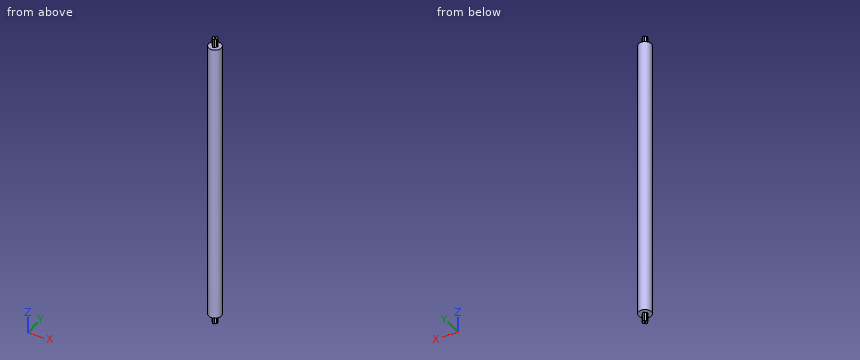
```python
from build123d import *

# Parameters (mm, degrees)
F0_R     = 22.5
F1_DEPTH = 1000
F4_DEPTH = 31
F5_R     = 2.5
F6_DEPTH = 40
F7_DEPTH = 30
F8_R     = 2.5
F9_DEPTH = 30


with BuildPart() as f1:
    # F0 (on Top) → F1 (new body)
    with BuildSketch(Plane.XY):
        Circle(F0_R)
    extrude(amount=F1_DEPTH)

    # F3 (on face) → F4 (join)
    with BuildSketch(Plane(origin=(0, 0, 0), x_dir=(1, 0, 0), z_dir=(0, 0, -1))):
        with BuildLine():
            ThreePointArc((7.0710678119, 2.5), (7.3919891974, 1.2682648404), (7.5, 0))
            ThreePointArc((7.5, 0), (7.3919069765, -1.268743966), (7.0707436663, -2.500916633))
            Line((7.0707436663, -2.500916633), (9.7997435124, -2.5))
            Line((9.7997435124, -2.5), (9.7997435124, 0))
            Line((9.7997435124, 0), (9.7997435124, 2.5))
            Line((9.7997435124, 2.5), (7.0710678119, 2.5))
        make_face()
        with BuildLine():
            Line((2.5, -9.7997435124), (2.5, -7.0710678119))
            ThreePointArc((2.5, -7.0710678119), (-0.0004861292, -7.4999999842), (-2.500916633, -7.0707436663))
            Line((-2.500916633, -7.0707436663), (-2.5, -9.7997435124))
            Line((-2.5, -9.7997435124), (0, -9.7997435124))
            Line((0, -9.7997435124), (2.5, -9.7997435124))
        make_face()
        with BuildLine():
            ThreePointArc((-7.0710678119, -2.5), (-7.4999999842, 0.0004861292), (-7.0707436663, 2.500916633))
            Line((-7.0707436663, 2.500916633), (-9.7997435124, 2.5))
            Line((-9.7997435124, 2.5), (-9.7997435124, 0))
            Line((-9.7997435124, 0), (-9.7997435124, -2.5))
            Line((-9.7997435124, -2.5), (-7.0710678119, -2.5))
        make_face()
        with BuildLine():
            ThreePointArc((7.0707436663, -2.500916633), (7.3919069765, -1.268743966), (7.5, 0))
            ThreePointArc((7.5, 0), (7.3919891974, 1.2682648404), (7.0710678119, 2.5))
            ThreePointArc((7.0710678119, 2.5), (5.303644593, 5.3029571025), (2.500916633, 7.0707436663))
            ThreePointArc((2.500916633, 7.0707436663), (0.0004861292, 7.4999999842), (-2.5, 7.0710678119))
            ThreePointArc((-2.5, 7.0710678119), (-5.3029571025, 5.303644593), (-7.0707436663, 2.500916633))
            ThreePointArc((-7.0707436663, 2.500916633), (-7.4999999842, 0.0004861292), (-7.0710678119, -2.5))
            ThreePointArc((-7.0710678119, -2.5), (-5.303644593, -5.3029571025), (-2.500916633, -7.0707436663))
            ThreePointArc((-2.500916633, -7.0707436663), (-0.0004861292, -7.4999999842), (2.5, -7.0710678119))
            ThreePointArc((2.5, -7.0710678119), (5.3029571025, -5.303644593), (7.0707436663, -2.500916633))
        make_face()
        with BuildLine():
            ThreePointArc((-2.5, 7.0710678119), (0.0004861292, 7.4999999842), (2.500916633, 7.0707436663))
            Line((2.500916633, 7.0707436663), (2.5, 9.7997435124))
            Line((2.5, 9.7997435124), (0, 9.7997435124))
            Line((0, 9.7997435124), (-2.5, 9.7997435124))
            Line((-2.5, 9.7997435124), (-2.5, 7.0710678119))
        make_face()
    extrude(amount=F4_DEPTH)

    # F5 (on face) → F6 (cut)
    with BuildSketch(Plane(origin=(0, 0, -31), x_dir=(1, 0, 0), z_dir=(0, 0, -1))):
        Circle(F5_R)
    extrude(amount=-F6_DEPTH, mode=Mode.SUBTRACT)

    # F2 (on face) → F7 (join)
    with BuildSketch(Plane.XY.offset(1000)):
        with BuildLine():
            ThreePointArc((7.0707436663, -2.500916633), (7.3919069765, -1.268743966), (7.5, 0))
            ThreePointArc((7.5, 0), (7.3919891974, 1.2682648404), (7.0710678119, 2.5))
            ThreePointArc((7.0710678119, 2.5), (5.303644593, 5.3029571025), (2.500916633, 7.0707436663))
            ThreePointArc((2.500916633, 7.0707436663), (0.0004861292, 7.4999999842), (-2.5, 7.0710678119))
            ThreePointArc((-2.5, 7.0710678119), (-5.3029571025, 5.303644593), (-7.0707436663, 2.500916633))
            ThreePointArc((-7.0707436663, 2.500916633), (-7.4999999842, 0.0004861292), (-7.0710678119, -2.5))
            ThreePointArc((-7.0710678119, -2.5), (-5.303644593, -5.3029571025), (-2.500916633, -7.0707436663))
            ThreePointArc((-2.500916633, -7.0707436663), (-0.0004861292, -7.4999999842), (2.5, -7.0710678119))
            ThreePointArc((2.5, -7.0710678119), (5.3029571025, -5.303644593), (7.0707436663, -2.500916633))
        make_face()
        with BuildLine():
            ThreePointArc((-7.0710678119, -2.5), (-7.4999999842, 0.0004861292), (-7.0707436663, 2.500916633))
            Line((-7.0707436663, 2.500916633), (-9.7997435124, 2.5))
            Line((-9.7997435124, 2.5), (-9.7997435124, 0))
            Line((-9.7997435124, 0), (-9.7997435124, -2.5))
            Line((-9.7997435124, -2.5), (-7.0710678119, -2.5))
        make_face()
        with BuildLine():
            ThreePointArc((-2.5, 7.0710678119), (0.0004861292, 7.4999999842), (2.500916633, 7.0707436663))
            Line((2.500916633, 7.0707436663), (2.5, 9.7997435124))
            Line((2.5, 9.7997435124), (0, 9.7997435124))
            Line((0, 9.7997435124), (-2.5, 9.7997435124))
            Line((-2.5, 9.7997435124), (-2.5, 7.0710678119))
        make_face()
        with BuildLine():
            ThreePointArc((7.0710678119, 2.5), (7.3919891974, 1.2682648404), (7.5, 0))
            ThreePointArc((7.5, 0), (7.3919069765, -1.268743966), (7.0707436663, -2.500916633))
            Line((7.0707436663, -2.500916633), (9.7997435124, -2.5))
            Line((9.7997435124, -2.5), (9.7997435124, 0))
            Line((9.7997435124, 0), (9.7997435124, 2.5))
            Line((9.7997435124, 2.5), (7.0710678119, 2.5))
        make_face()
        with BuildLine():
            Line((2.5, -9.7997435124), (2.5, -7.0710678119))
            ThreePointArc((2.5, -7.0710678119), (-0.0004861292, -7.4999999842), (-2.500916633, -7.0707436663))
            Line((-2.500916633, -7.0707436663), (-2.5, -9.7997435124))
            Line((-2.5, -9.7997435124), (0, -9.7997435124))
            Line((0, -9.7997435124), (2.5, -9.7997435124))
        make_face()
    extrude(amount=F7_DEPTH)

    # F8 (on face) → F9 (cut)
    with BuildSketch(Plane.XY.offset(1030)):
        Circle(F8_R)
    extrude(amount=-F9_DEPTH, mode=Mode.SUBTRACT)


solid = f1.part
```
Here's how the part is built. I have some questions about the finished solid (model axes, mm). Round coordinates to 2 decimals unless told otherwise and drop trailing zeros. Write each loop counter-clockwise with the first axis right and the second up, starting at its lowest first coordinate (ties: lowest second). Pieces come first, ordered by that corner, then holes.
Q1. Please list where these lines run through material, in increasing order: probe 1 along Y at (x, z) = (0, -4.5); probe 2 along Z at (x, y) = (-11, -8.5).
Q2. Will these pins go through, and if not, where does the flat tip stop? P1, Ø8, axis at y = 4.5, z = 718, coming from the +X side; P2, Ø2, axis at x = 18, z = 265.5, coming from the +Y side; P3, Ø12, axis at x = -16.5, z = 76.5, coming from the +Y side.
Q3. If we section it at A-A on z = 819.5: Write out the boundary of the cut face in (x, y).
Answer below:
1. probe 1: y = -9.8 to -2.5, 2.5 to 9.8
1. probe 2: z = 0 to 1000
2. P1: stops at x = 22.49
2. P2: stops at y = 14.74
2. P3: stops at y = 19.9
3. outline: circle Ø45 at (0, 0)
